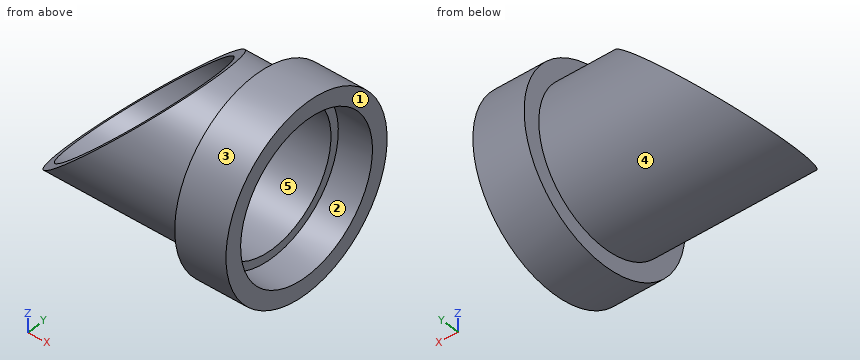
from build123d import *

# Parameters (mm, degrees)
SKETCH3_R                = 57.15
SKETCH3_R_2              = 50.8
BOSS_EXTRUDE2_DEPTH      = 152.4
BOSS_EXTRUDE3_DEPTH      = 25.4
BOSS_EXTRUDE3_DEPTH_BACK = 12.7
SKETCH4_R                = 69.85
SKETCH4_R_2              = 57.15
CUT_EXTRUDE1_DEPTH       = 127
CUT_EXTRUDE1_DEPTH_BACK  = 127


with BuildPart() as part:
    # Sketch3 → Boss-Extrude2 (new body)
    with BuildSketch(Plane(origin=(0, 0, 0), x_dir=(0, 0, -1), z_dir=(1, 0, 0))):
        with Locations(Location((0, 0, 0), (0, 0, 180))):
            Circle(SKETCH3_R)
        with Locations(Location((0, 0, 0), (0, 0, 180))):
            Circle(SKETCH3_R_2, mode=Mode.SUBTRACT)
    extrude(amount=BOSS_EXTRUDE2_DEPTH)

    # Sketch4 → Boss-Extrude3 (add, two sides: drawn at the far end of the back side and taken through both)
    with BuildSketch(Plane(origin=(152.4, 0, 0), x_dir=(0, 0, -1), z_dir=(1, 0, 0)).offset(-BOSS_EXTRUDE3_DEPTH_BACK)):
        Circle(SKETCH4_R)
        with Locations(Location((0, 0, 0), (0, 0, 180))):
            Circle(SKETCH4_R_2, mode=Mode.SUBTRACT)
    extrude(amount=BOSS_EXTRUDE3_DEPTH + BOSS_EXTRUDE3_DEPTH_BACK)

    # Sketch5 → Cut-Extrude1 (cut, two sides: drawn at the far end of the back side and taken through both)
    with BuildSketch(Plane(origin=(0, 0, 0), x_dir=(1, 0, 0), z_dir=(0, 1, 0)).offset(-CUT_EXTRUDE1_DEPTH_BACK)):
        Polygon((0, -57.15), (114.3, -57.15), (0, 57.15), align=None)
    extrude(amount=CUT_EXTRUDE1_DEPTH + CUT_EXTRUDE1_DEPTH_BACK, mode=Mode.SUBTRACT)


solid = part.part
Design review of the part built by this model. Coordinates are the model's own, in mm. Face numbers are marked on the shaded views. A direction names the side the tool comes from. Round coordinates to 2 decimals unless told otherwise and drop trailing zeros. Order: outer loops, then holes, each group sorted by start corner. A loop starts at its lowest first (then second) coordinate and runs counter-clockwise, first axis right, second up.
1) Machinability: for the marked faces 4 and 5, which of the approach directions +Z, -Z, +X, -X, +Y, -Y give a long, thin tool a straight path to every point of the face, cutting with its end or side? Answer none if there is none.
The answers:
face 4: -X
face 5: +X, -X
2) Consider section A-A (y = 0). State the section outline as (x, z) points, plus the area to 3 significant figures.
The answers:
outline: (0, -57.15) - (139.7, -57.15) - (139.7, -69.85) - (177.8, -69.85) - (177.8, -57.15) - (152.4, -57.15) - (152.4, -50.8) - (6.35, -50.8) - close; (107.95, 50.8) - (152.4, 50.8) - (152.4, 57.15) - (177.8, 57.15) - (177.8, 69.85) - (139.7, 69.85) - (139.7, 57.15) - (114.3, 57.15) - close
area: 2,180 mm2
3) Consider section C-C (x = 43). State the section outline as (y, z) points.
The answers:
outline: (-55.37, -14.15) arc R57.15 ccw to (55.37, -14.15) - (48.79, -14.15) arc R50.8 cw to (-48.79, -14.15) - close
4) Clearance check with flat-ended pins moving along their axes: pin 1 Ø1.5 at (x, y) = (141, -11) entering from -Z; pin 2 Ø5 at (x, y) = (112.5, 49) entering from -Z; pin 3 Ø5 at (x, y) = (75.5, -7) entering from +Z. State where each tip first meets the part, or that it passes through.
The answers:
pin 1: stops at z = -69.09
pin 2: stops at z = -33.22
pin 3: stops at z = -49.9
5) Consider section B-B (z = 0). State the section outline as (x, y) points, plus the area to 3 significant figures.
The answers:
outline: (57.15, -57.15) - (139.7, -57.15) - (139.7, -69.85) - (177.8, -69.85) - (177.8, -57.15) - (152.4, -57.15) - (152.4, -50.8) - (57.15, -50.8) - close; (57.15, 50.8) - (152.4, 50.8) - (152.4, 57.15) - (177.8, 57.15) - (177.8, 69.85) - (139.7, 69.85) - (139.7, 57.15) - (57.15, 57.15) - close
area: 2,180 mm2
6) Draft analysis for pull direction Y (two halves, no side actions). For the marked faces 1, 2 and 3, state which applies: released by +Y, released by -Y, zero draft, split by the parting line, or undercut.
The answers:
face 1: zero draft
face 2: undercut
face 3: split by the parting line
7) Consider section D-D (z = -61). State the section outline as (x, y) points.
The answers:
outline: (139.7, -34.03) - (177.8, -34.03) - (177.8, 34.03) - (139.7, 34.03) - close
8) For L1, parallel to Y at x = 160, z = 0; L2, parallel to Y at x = 102, z = 0; L3, parallel to Z at x = 96, y = 0, list the stretches that pass through material, from the lowest coordinate up.
The answers:
L1: y = -69.85 to -57.15, 57.15 to 69.85
L2: y = -57.15 to -50.8, 50.8 to 57.15
L3: z = -57.15 to -50.8
